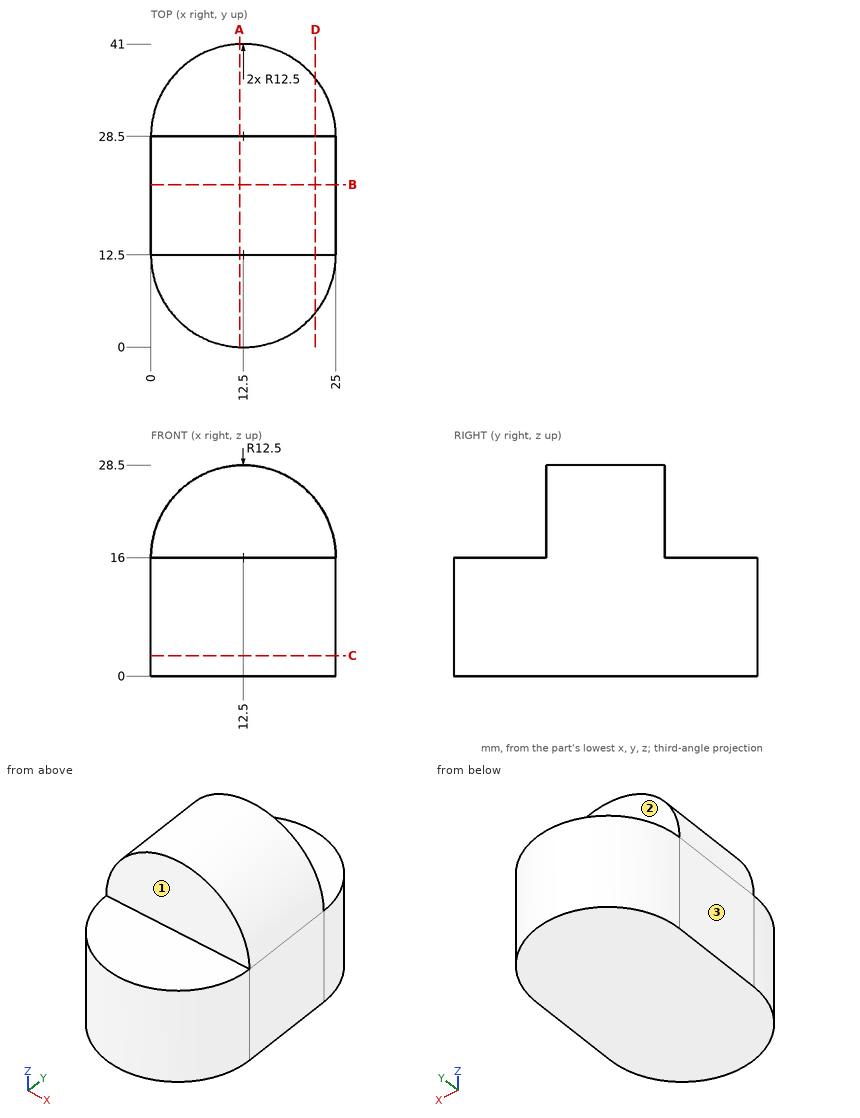
Print and shaded views of the part. All mm, measured from the part's lowest x, y and z. A direction names the side the tool comes from. Coordinates: 2 decimals unless noted, no trailing zeros. Order: outer loops, then holes, each group sorted by start corner. A loop starts at its lowest first (then second) coordinate and runs counter-clockwise, first axis right, second up. Notation, with made-up numbers: (-39, -27) -> (-20, -27) arc R25 cw to (-20, -2) -> close; hole circle Ø10 at (-39.75, 59.25). An arc over 180 degrees is marked (long way). Answer as a JSON object with one key per item and string values. Group by question number.
1) Drill centre lines: L1, parallel to Z at x = 3.25, y = 32; L2, parallel to Y at x = 18, z = 20.5; L3, parallel to X at y = 33.5, z = 1.5. Where is each one in solid material? Low to high.
2) Cut at A-A, the plane x = 12. Write the cut outline in (y, z).
3) Flat gauge pins, fed straight in: pin 1 (12 mm diameter, centred on x = 13, z = 23, fed in from +Y); pin 2 (14 mm diameter, centred on x = 13, y = 36.5, fed in from +Z); pin 3 (8 mm diameter, centred on x = 17, z = 12, fed in from -Y). Where does each tip first touch, or does it go through?
4) Cut at C-C, the plane z = 2.75. Write the cut outline in (x, y).
5) Cut at D-D, the plane x = 22.25. Write the cut outline in (y, z).
6) Cut at B-B, the plane y = 22. Write the cut outline in (x, z).
7) Which spindle directions (+Z, -Z, +X, -X, +Y, -Y) get a long thin tool onto all of the face, cutting with end or side? Do the marked faces 1, 2 and 3. Say none if no direction does.
Check values:
{
 "1": {"L1": "z = 0 to 16", "L2": "y = 12.5 to 28.5", "L3": "x = 1.04 to 23.96"},
 "2": {"outline": "(0.01, 0) -> (40.99, 0) -> (40.99, 16) -> (28.5, 16) -> (28.5, 28.49) -> (12.5, 28.49) -> (12.5, 16) -> (0.01, 16) -> close"},
 "3": {"pin 1": "stops at y = 28.5", "pin 2": "stops at z = 16", "pin 3": "stops at y = 0.01"},
 "4": {"outline": "(0, 12.5) arc R12.5 ccw to (25, 12.5) -> (25, 28.5) arc R12.5 ccw to (0, 28.5) -> close"},
 "5": {"outline": "(4.68, 0) -> (36.32, 0) -> (36.32, 16) -> (28.5, 16) -> (28.5, 23.82) -> (12.5, 23.82) -> (12.5, 16) -> (4.68, 16) -> close"},
 "6": {"outline": "(0, 0) -> (25, 0) -> (25, 16) arc R12.5 ccw to (0, 16) -> close"},
 "7": {"face 1": "+Z, +X, -X, -Y", "face 2": "+Z, +X, -X, +Y", "face 3": "+Z, -Z, -X, +Y, -Y"}
}
